Geometry: final body of the model. Coordinates: model frame, mm. A direction names the side the tool comes from. Round coordinates to 2 decimals unless told otherwise and drop trailing zeros. Loops run counter-clockwise (first coordinate to the right, second up) from the corner with the lowest first, then second, coordinate; pieces in that order, holes last. Notation, with made-up numbers: (-26, 64) - (-11, 64) arc R18 ccw to (-11, 84) - close; hole circle Ø4 at (39.5, 53). An arc over 180 degrees is marked (long way). Return JSON: item names as keys, results as strings. Group by question number.
1. Material intervals for probe 1 along Z at (x, y) = (34, 43); probe 2 along Y at (x, z) = (0.5, -23); probe 3 along Y at (x, z) = (0, 3), sorted ascending.
2. Section D-D on x = 47. Return loops of the section in (y, z), and give its area (4 significant figures).
3. Section B-B on y = 44.5. Return loops of the section in (x, z).
4. Section A-A on z = 29. Return loops of the section in (x, y), and give its area (3 significant figures).
5. First-contact query: pin 1 Ø3 at (x, z) = (-1.5, 25) entering from -Y; pin 2 Ø12 at (x, z) = (-40, -13) entering from +Y; pin 3 Ø10 at (x, z) = (18.5, -13) entering from -Y. Flat tips, straight axial feed; report the tip coordinate or a pass-through.
6. Draft query along Y for faces 5 (the face through (-30, 46, 2)), 6 (the face through (13.38, -25.73, 23.3)), 7 (the face through (-43.25, -33.16, 0.03)). Return one class per face: +Y half, -Y half, draft (parallel to the pull), parting line (faces both ways), or undercut.
7. Section C-C on x = -33.5. Return loops of the section in (y, z).
8. Set-up query: faces 1 (the face through (29, -3, 38)), 2 (the face through (5.077, 38.668, 24.818)), 3 (the face through (28, -21, -25)), 4 (the face through (-13, -37, -12)). Return all of +Z, -Z, +X, -X, +Y, -Y with unobstructed straight access to the full face (end or side cutting, diameter ignored); none if empty.
from build123d import *

# Parameters (mm, degrees)
SKETCH_1_R               = 56.5
EXTRUDE_1_DEPTH          = 12
EXTRUDE_1_DEPTH_BACK     = 12
SKETCH_2_R               = 74.899602785
SKETCH_2_R_2             = 54.5
CUT_EXTRUDE_1_DEPTH      = 2
CUT_EXTRUDE_1_DEPTH_BACK = 2
SKETCH_3_R               = 39
EXTRUDE_2_DEPTH          = 26
SKETCH_4_R               = 52.483360518
SKETCH_4_R_2             = 35
CUT_EXTRUDE_2_DEPTH      = 3
CUT_EXTRUDE_2_DEPTH_BACK = 3
SKETCH_5_R               = 27.5
CUT_EXTRUDE_3_DEPTH      = 80
SKETCH_6_R               = 29
CUT_EXTRUDE_4_DEPTH      = 50


with BuildPart() as part:
    # Sketch 1 → Extrude 1 (new body, two sides)
    with BuildSketch(Plane.XY) as extrude_1_sk:
        Circle(SKETCH_1_R)
    extrude(amount=EXTRUDE_1_DEPTH)
    extrude(extrude_1_sk.sketch, amount=-EXTRUDE_1_DEPTH_BACK)

    # Sketch 2 → Cut-Extrude 1 (cut, two sides)
    with BuildSketch(Plane.XY) as cut_extrude_1_sk:
        Circle(SKETCH_2_R)
        Circle(SKETCH_2_R_2, mode=Mode.SUBTRACT)
    extrude(amount=CUT_EXTRUDE_1_DEPTH, mode=Mode.SUBTRACT)
    extrude(cut_extrude_1_sk.sketch, amount=-CUT_EXTRUDE_1_DEPTH_BACK, mode=Mode.SUBTRACT)

    # Sketch 3 → Extrude 2 (add)
    with BuildSketch(Plane(origin=(0, 0, -12), x_dir=(-1, 0, 0), z_dir=(0, 0, -1))):
        Circle(SKETCH_3_R)
    extrude_2 = extrude(amount=EXTRUDE_2_DEPTH)

    # Mirror 1: Extrude 2 across plane
    add(extrude_2.mirror(Plane.XY))

    # Sketch 4 → Cut-Extrude 2 (cut, two sides)
    with BuildSketch(Plane(origin=(0, 0, -25), x_dir=(-1, 0, 0), z_dir=(0, 0, -1))) as cut_extrude_2_sk:
        Circle(SKETCH_4_R)
        Circle(SKETCH_4_R_2, mode=Mode.SUBTRACT)
    extrude(amount=CUT_EXTRUDE_2_DEPTH, mode=Mode.SUBTRACT)
    extrude(cut_extrude_2_sk.sketch, amount=-CUT_EXTRUDE_2_DEPTH_BACK, mode=Mode.SUBTRACT)

    # Sketch 5 → Cut-Extrude 3 (cut)
    with BuildSketch(Plane.XY.offset(38)):
        Circle(SKETCH_5_R)
    extrude(amount=-CUT_EXTRUDE_3_DEPTH, mode=Mode.SUBTRACT)

    # Sketch 6 → Cut-Extrude 4 (cut)
    with BuildSketch(Plane.XY.offset(9)):
        Circle(SKETCH_6_R)
    cut_extrude_4 = extrude(amount=CUT_EXTRUDE_4_DEPTH, mode=Mode.SUBTRACT)

    # Mirror 2: Cut-Extrude 4 across plane
    add(cut_extrude_4.mirror(Plane.XY), mode=Mode.SUBTRACT)


solid = part.part
Taken from the geometry:
{
 "1": {"probe 1": "-12 to -2, 2 to 12", "probe 2": "-35 to -29, 29 to 35", "probe 3": "-56.5 to -27.5, 27.5 to 56.5"},
 "2": {"outline": "(-31.36, -12) - (31.36, -12) - (31.36, -2) - (27.59, -2) - (27.59, 2) - (31.36, 2) - (31.36, 12) - (-31.36, 12) - (-31.36, 2) - (-27.59, 2) - (-27.59, -2) - (-31.36, -2) - close", "area": "1,475 mm2"},
 "3": {"outline": "(-34.81, -12) - (34.81, -12) - (34.81, -2) - (31.46, -2) - (31.46, 2) - (34.81, 2) - (34.81, 12) - (-34.81, 12) - (-34.81, 2) - (-31.46, 2) - (-31.46, -2) - (-34.81, -2) - close"},
 "4": {"outline": "circle Ø78 at (0, 0); hole circle Ø58 at (0, 0)", "area": "2,140 mm2"},
 "5": {"pin 1": "y = -39", "pin 2": "y = 45.06", "pin 3": "y = -54.84"},
 "6": {"face 5": "draft", "face 6": "undercut", "face 7": "parting line"},
 "7": {"outline": "(-45.5, -12) - (-19.97, -12) - (-19.97, -22) - (-10.14, -22) - (-10.14, -28) - (-19.97, -28) - (-19.97, -38) - (19.97, -38) - (19.97, -28) - (10.14, -28) - (10.14, -22) - (19.97, -22) - (19.97, -12) - (45.5, -12) - (45.5, -2) - (42.99, -2) - (42.99, 2) - (45.5, 2) - (45.5, 12) - (19.97, 12) - (19.97, 38) - (-19.97, 38) - (-19.97, 12) - (-45.5, 12) - (-45.5, 2) - (-42.99, 2) - (-42.99, -2) - (-45.5, -2) - close"},
 "8": {"face 1": "+Z, +X, -X, +Y, -Y", "face 2": "+Z", "face 3": "none", "face 4": "-Z"}
}
